from build123d import *

# Parameters (mm, degrees)
BOSS_EXTRUDE1_DEPTH = 10
CUT_EXTRUDE1_DEPTH  = 8
SKETCH6_R           = 1.5
CUT_EXTRUDE2_DEPTH  = 12
FILLET1_R           = 1
BOSS_EXTRUDE2_DEPTH = 2
FILLET2_R           = 0.5


with BuildPart() as part:
    # Sketch4 → Boss-Extrude1 (new body)
    with BuildSketch(Plane.XY):
        with BuildLine():
            Line((1, 0.1), (11, 0.1))
            ThreePointArc((11, 0.1), (11.707106781, 0.392893219), (12, 1.1))
            Line((12, 1.1), (12, 11.9))
            ThreePointArc((12, 11.9), (11.707106781, 12.607106781), (11, 12.9))
            Line((11, 12.9), (1, 12.9))
            ThreePointArc((1, 12.9), (0.292893219, 12.607106781), (0, 11.9))
            Line((0, 11.9), (0, 1.1))
            ThreePointArc((0, 1.1), (0.292893219, 0.392893219), (1, 0.1))
        make_face()
    extrude(amount=BOSS_EXTRUDE1_DEPTH)

    # Sketch5 → Cut-Extrude1 (cut)
    with BuildSketch(Plane.XY.offset(10)):
        with BuildLine():
            Line((11.445, 6.5), (10.555, 6.5))
            ThreePointArc((10.555, 6.5), (10, 5.945), (9.445, 6.5))
            Line((9.445, 6.5), (8.555, 6.5))
            ThreePointArc((8.555, 6.5), (8, 5.945), (7.445, 6.5))
            Line((7.445, 6.5), (6.555, 6.5))
            ThreePointArc((6.555, 6.5), (6, 5.945), (5.445, 6.5))
            Line((5.445, 6.5), (4.555, 6.5))
            ThreePointArc((4.555, 6.5), (4, 5.945), (3.445, 6.5))
            Line((3.445, 6.5), (2.555, 6.5))
            ThreePointArc((2.555, 6.5), (2, 5.945), (1.445, 6.5))
            Line((1.445, 6.5), (0.555, 6.5))
            ThreePointArc((0.555, 6.5), (0.392444264, 6.107555736), (0, 5.945))
            Line((0, 5.945), (0, 7.345))
            Line((0, 7.345), (12, 7.345))
            Line((12, 7.345), (12, 5.945))
            ThreePointArc((12, 5.945), (11.607555736, 6.107555736), (11.445, 6.5))
        make_face()
    extrude(amount=-CUT_EXTRUDE1_DEPTH, mode=Mode.SUBTRACT)

    # Sketch6 → Cut-Extrude2 (cut)
    with BuildSketch(Plane.ZY):
        with Locations((6, 3.25)):
            Circle(SKETCH6_R)
        Polygon((2, 2.65), (2, 0.1), (0, 0.1), (0, 2.15), align=None)
        Polygon((0, 12.9), (0, 10.85), (2, 10.35), (2, 12.9), align=None)
    extrude(amount=-CUT_EXTRUDE2_DEPTH, mode=Mode.SUBTRACT)

    # Fillet1
    fillet1_edges = [part.edges().sort_by_distance(p)[0] for p in [
        (6, 7.345, 10),
    ]]
    fillet(fillet1_edges, radius=FILLET1_R)

    # Sketch7 → Boss-Extrude2 (add)
    with BuildSketch(Plane.ZY):
        Polygon((7.876388375, 1.1), (9.117691454, 3.25), (7.879275126, 5.395), (10, 5.395), (10, 1.1), align=None)
        Polygon((2, 1.1), (2, 5.395), (4.120724874, 5.395), (2.882308546, 3.25), (4.123611625, 1.1), align=None)
    extrude(amount=BOSS_EXTRUDE2_DEPTH)

    # Fillet2
    fillet2_edges = [part.edges().sort_by_distance(p)[0] for p in [
        (12, 2.4, 1),
        (0, 10.6, 1),
        (12, 10.6, 1),
        (0, 2.4, 1),
    ]]
    fillet(fillet2_edges, radius=FILLET2_R)


solid = part.part
Check sheet for the modelled part. Datum: model origin and axes. Units: mm. A direction names the side the tool comes from. Give positions to 0.01 mm unless a question says otherwise; leave off trailing zeros. Write each loop counter-clockwise with the first axis right and the second up, starting at its lowest first coordinate (ties: lowest second). Pieces come first, ordered by that corner, then holes. Notation, with made-up numbers: (14, 4.5) -> (26, 4.5) arc R23 cw to (26, 13.5) -> close; hole circle Ø11 at (35, -7.75). An arc over 180 degrees is marked (long way). Use one line per item in the form item = value. Start each with the question number.
1. Section check B-B (x = 4). Record the cut outline in (y, z) (3 decimals), and give its area (3 significant figures).
2. Section check D-D (y = 3.75). Record the cut outline in (x, z), and give its area (3 significant figures).
3. Access from +Z, -Z, +X, -X, +Y, -Y to the whole of each face (thin tool, end or side, straight path). Record for faces 4 (the flat face through (5.9, 2.4, 1)), 5 (the cylindrical face through (8.012, 5.945, 6.056)), 6 (the cylindrical face through (0.143, 10.435, 1.039)), 7 (the cylindrical face through (6.08, 7.63, 9.7)), 8 (the cylindrical face through (11.85, 2.56, 1.04)).
4. Mould release check, pull along X, two halves, no side actions. Record for faces 1 (the flat face through (-1, 1.1, 3)), 2 (the cylindrical face through (0.143, 2.565, 1.039)), 3 (the cylindrical face through (4.012, 5.945, 6.056)): pulls with the +X half, pulls with the -X half, needs draft (parallel to the pull), parting line crosses it, or undercut.
5. Section check A-A (z = 6). Record the cut outline in (x, y) (3 decimals).
6. Go/stop test with flat-tipped pins: P1, Ø5, axis at y = 3.25, z = 6, coming from the -X side; P2, Ø1, axis at x = -1, z = 2.5, coming from the +Y side (3 decimals); P3, Ø0.6, axis at x = -1, z = 8.5, coming from the -Y side. Record where each tip stops, or that it passes through.
7. Thickness scan on line 1 along Y through (x, z) = (9, 6) (3 decimals); line 2 along Y through (x, z) = (10, 2.5) (3 decimals); line 3 along X through (y, z) = (6.25, 3). Record the ranges inside material, lowest first. Write a range as from..to.
Conclusion:
q1.outline = (0.1, 2) -> (2.65, 2) -> (2.15, 0) -> (10.85, 0) -> (10.35, 2) -> (12.9, 2) -> (12.9, 10) -> (8.345, 10) arc R1 ccw to (7.345, 9) -> (7.345, 2) -> (5.945, 2) -> (5.945, 10) -> (0.1, 10) -> close; hole circle Ø3 at (3.25, 6)
q1.area = 100 mm²
q2.outline = (-2, 2) -> (0, 2) -> (0, 0) -> (12, 0) -> (12, 4.59) -> (0, 4.59) -> (0, 3.17) -> (-2, 3.17) -> close; (-2, 8.83) -> (0, 8.83) -> (0, 7.41) -> (12, 7.41) -> (12, 10) -> (-2, 10) -> close
q2.area = 90.7 mm²
q3.face_4 = +X, -X, -Y
q3.face_5 = +Z
q3.face_6 = -X, +Y
q3.face_7 = +Z, +X, -X
q3.face_8 = +X, -Y
q4.face_1 = needs draft
q4.face_2 = pulls with the -X half
q4.face_3 = undercut
q5.outline = (0, 1.1) arc R1 ccw to (1, 0.1) -> (11, 0.1) arc R1 ccw to (12, 1.1) -> (12, 1.75) -> (0, 1.75) -> close; (0, 4.75) -> (12, 4.75) -> (12, 5.945) arc R0.555 cw to (11.445, 6.5) -> (10.555, 6.5) arc R0.555 cw to (9.445, 6.5) -> (8.555, 6.5) arc R0.555 cw to (7.445, 6.5) -> (6.555, 6.5) arc R0.555 cw to (5.445, 6.5) -> (4.555, 6.5) arc R0.555 cw to (3.445, 6.5) -> (2.555, 6.5) arc R0.555 cw to (1.445, 6.5) -> (0.555, 6.5) arc R0.555 cw to (0, 5.945) -> close; (0, 7.345) -> (12, 7.345) -> (12, 11.9) arc R1 ccw to (11, 12.9) -> (1, 12.9) arc R1 ccw to (0, 11.9) -> close
q6.P1 = 0
q6.P2 = 5.395
q6.P3 = 1.1
q7.line_1 = 0.1..1.75, 4.75..6.5, 7.345..12.9
q7.line_2 = 0.1..5.945, 7.345..12.9
q7.line_3 = 0.5..1.5, 2.5..3.5, 4.5..5.5, 6.5..7.5, 8.5..9.5, 10.5..11.5
